from build123d import *

# Parameters (mm, degrees)
CUT_EXTRUDE2_DEPTH   = 23.368
M3_CLEARANCE_HOLE1_D = 3.6
SKETCH10_OUTSIDE_W   = 29.468
SKETCH10_OUTSIDE_H   = 29.468
SKETCH10_OUTSIDE_R   = 4.953
CUT_EXTRUDE3_DEPTH   = 30.033261092


with BuildPart() as part:
    # Sketch1 → Revolve1 (revolve)
    with BuildSketch(Plane(origin=(0, 0, 0), x_dir=(0, 0, -1), z_dir=(1, 0, 0))):
        Polygon((0, 25.4), (9.9441, 25.4), (9.9441, 23.368), (4.953, 23.368), (4.953, 0), (0, 0), align=None)
    revolve(axis=Axis((0, 0, 0), (0, 1, 0)))

    # Sketch4 → Cut-Extrude2 (cut)
    with BuildSketch(Plane.XZ):
        Polygon((1.613116652, -2.794), (3.226233304, 0), (1.613116652, 2.794), (-1.613116652, 2.794), (-3.226233304, 0), (-1.613116652, -2.794), align=None)
    extrude(amount=-CUT_EXTRUDE2_DEPTH, mode=Mode.SUBTRACT)

    # M3 Clearance Hole1 (through all)
    with Locations(Plane(origin=(0, 25.4, 0), x_dir=(1, 0, 0), z_dir=(0, 1, 0))):
        with Locations((-6.985, 0), (0, 0), (6.985, 0), (0, 6.985), (0, -6.985)):
            Hole(M3_CLEARANCE_HOLE1_D / 2)

    # Sketch10 outside → Cut-Extrude3 (cut, through all)
    with BuildSketch(Plane.XZ):
        Rectangle(SKETCH10_OUTSIDE_W, SKETCH10_OUTSIDE_H)
        with Locations(Location((0, 0, 0), (0, 0, 270))):
            Circle(SKETCH10_OUTSIDE_R, mode=Mode.SUBTRACT)
    extrude(amount=-CUT_EXTRUDE3_DEPTH, mode=Mode.SUBTRACT)


solid = part.part
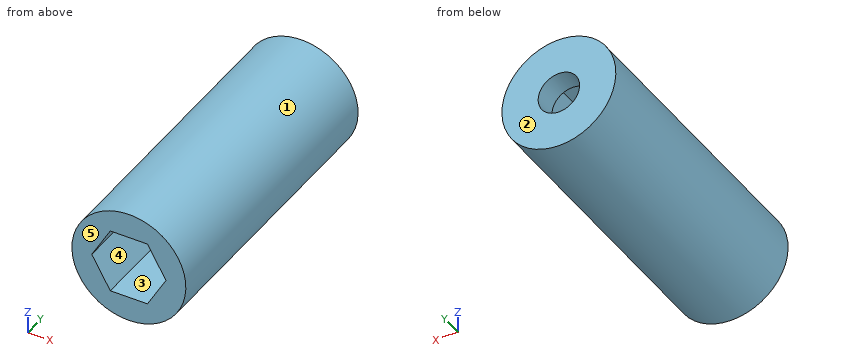
CAD build for the part. Positions are in the model's coordinates, mm. Face numbers are marked on the shaded views. A direction names the side the tool comes from. Coordinates: 2 decimals unless noted, no trailing zeros. Loops run counter-clockwise (first coordinate to the right, second up) from the corner with the lowest first, then second, coordinate; pieces in that order, holes last. Notation, with made-up numbers: (23, -30.75) -> (36, -30.75) arc R14 ccw to (36, -17.75) -> close; hole circle Ø7 at (3, 37). An arc over 180 degrees is marked (long way). One line per item, written item: value.
1. Slice it at D-D on z = -3.5. Write the cut outline in (x, y), and give its area (3 significant figures).
Answers:
outline: (-3.5, 0) -> (3.5, 0) -> (3.5, 25.4) -> (-3.5, 25.4) -> close
area: 178 mm^2
2. Slice it at C-C on z = -0.75. Write the cut outline in (x, y), and give its area (3 significant figures).
Answers:
outline: (-4.9, 0) -> (-2.79, 0) -> (-2.79, 23.37) -> (-1.64, 23.37) -> (-1.64, 25.4) -> (-4.9, 25.4) -> close; (1.64, 23.37) -> (2.79, 23.37) -> (2.79, 0) -> (4.9, 0) -> (4.9, 25.4) -> (1.64, 25.4) -> close
area: 112 mm^2
3. Drill centre lines: line 1 (Z direction, x = 0, y = 24.75); line 2 (Y direction, x = -2.75, z = 0.5); line 3 (Z direction, x = -2.25, y = 22.75). Where is each one in solid material? Low to high. Write a range as [from, to].
Answers:
line 1: z = [-4.95, -1.8], [1.8, 4.95]
line 2: y = [23.37, 25.4]
line 3: z = [-4.41, -1.69], [1.69, 4.41]
4. Which spindle directions (+Z, -Z, +X, -X, +Y, -Y) get a long thin tool onto all of the face, cutting with end or side? Do the marked faces 4 and 5. Say none if no direction does.
Answers:
face 4: -Y
face 5: +Z, -Z, +X, -X, -Y
5. Slice it at A-A on x = 0. Write the cut outline in (y, z).
Answers:
outline: (0, -4.95) -> (25.4, -4.95) -> (25.4, -1.8) -> (23.37, -1.8) -> (23.37, -2.79) -> (0, -2.79) -> close; (0, 2.79) -> (23.37, 2.79) -> (23.37, 1.8) -> (25.4, 1.8) -> (25.4, 4.95) -> (0, 4.95) -> close
6. Pull direction X, two halves, no side cores. Call the marked faces 1, 2 and 3: pulls with the +X half, pulls with the -X half, needs draft (parallel to the pull), parting line crosses it, or undercut.
Answers:
face 1: parting line crosses it
face 2: needs draft
face 3: undercut
7. Slice it at B-B on y = 8.75. Write the cut outline in (x, z), and give its area (3 significant figures).
Answers:
outline: circle Ø9.91 at (0, 0); hole (-3.23, 0) -> (-1.61, -2.79) -> (1.61, -2.79) -> (3.23, 0) -> (1.61, 2.79) -> (-1.61, 2.79) -> close
area: 50.0 mm^2
8. Flat gauge pins, fed straight in: P1, Ø3, axis at y = 13.5, z = 2, coming from the +X side; P2, Ø1.5, axis at x = -2.5, y = 20.5, coming from the -Z side. Where does each tip first touch, or does it go through?
Answers:
P1: stops at x = 4.93
P2: stops at z = -4.63
